from build123d import *

# Parameters (mm, degrees)
ESQUISSE1_W              = 200
ESQUISSE1_H              = 85
BOSS_EXTRU_1_DEPTH       = 30
ENL_V_MAT_EXTRU_3_DEPTH  = 28
ESQUISSE3_W              = 35
ESQUISSE3_H              = 85
ENL_V_MAT_EXTRU_4_DEPTH  = 18
ESQUISSE4_W              = 29.5
ESQUISSE4_H              = 80.5
ENL_V_MAT_EXTRU_5_DEPTH  = 10
CHANFREIN1_SIZE2         = 40
CHANFREIN1_SIZE          = 18
ENL_V_MAT_EXTRU_18_DEPTH = 220.374109685
ENL_V_MAT_EXTRU_19_DEPTH = 220.374109685
CHANFREIN5_SIZE2         = 30
CHANFREIN5_SIZE          = 40
CHANFREIN6_SIZE2         = 25
CHANFREIN6_SIZE          = 40
ESQUISSE10_W             = 40
ESQUISSE10_H             = 2
ENL_V_MAT_EXTRU_20_DEPTH = 2
ENL_V_MAT_EXTRU_21_DEPTH = 4
CONG_6_R                 = 6
CONG_7_R                 = 6
CHANFREIN7_SIZE2         = 119
CHANFREIN7_SIZE          = 2
CHANFREIN8_SIZE          = 0.47
CHANFREIN8_SIZE_2        = 28


# Some blends are built 0.0001 mm under size
with BuildPart() as part:
    # Esquisse1 → Boss.-Extru.1 (new body)
    with BuildSketch(Plane.XY):
        with Locations((100, 42.5)):
            Rectangle(ESQUISSE1_W, ESQUISSE1_H)
    extrude(amount=BOSS_EXTRU_1_DEPTH)

    # Esquisse2 → Enlèv. mat.-Extru.3 (cut)
    with BuildSketch(Plane.XY.offset(30)):
        Polygon((119.192122608, 49.886058148), (121.796845273, 35.113941852), (4.604722665, 14.44980871), (2, 29.221925005), align=None)
    extrude(amount=-ENL_V_MAT_EXTRU_3_DEPTH, mode=Mode.SUBTRACT)

    # Esquisse3 → Enlèv. mat.-Extru.4 (cut)
    with BuildSketch(Plane.XY.offset(30)):
        with Locations((182.5, 42.5)):
            Rectangle(ESQUISSE3_W, ESQUISSE3_H)
    extrude(amount=-ENL_V_MAT_EXTRU_4_DEPTH, mode=Mode.SUBTRACT)

    # Esquisse4 → Enlèv. mat.-Extru.5 (cut)
    with BuildSketch(Plane.XY.offset(12)):
        with Locations((183.25, 42)):
            Rectangle(ESQUISSE4_W, ESQUISSE4_H)
    extrude(amount=-ENL_V_MAT_EXTRU_5_DEPTH, mode=Mode.SUBTRACT)

    # Chanfrein1
    chanfrein1_edges = [part.edges().sort_by_distance(p)[0] for p in [
        (165, 42.5, 30),
    ]]
    chanfrein1_side = [part.faces().sort_by_distance(p)[0] for p in [
        (165, 42.5, 29.64),
    ]]
    chamfer(chanfrein1_edges, length=CHANFREIN1_SIZE - 0.0001, length2=CHANFREIN1_SIZE2 - 0.0001, reference=chanfrein1_side[0])  # a hair under: the kernel refuses the full size

    # Esquisse7 → Enlèv. mat.-Extru.18 (cut, through all)
    with BuildSketch(Plane.XY.offset(30)):
        Polygon((0, 37.959127411), (125, 60), (125, 85), (0, 85), align=None)
    extrude(amount=-ENL_V_MAT_EXTRU_18_DEPTH, mode=Mode.SUBTRACT)

    # Esquisse9 → Enlèv. mat.-Extru.19 (cut, through all)
    with BuildSketch(Plane.XY.offset(30)):
        Polygon((125, 30.113941852), (0, 8.073069264), (0, 0), (125, 0), align=None)
    extrude(amount=-ENL_V_MAT_EXTRU_19_DEPTH, mode=Mode.SUBTRACT)

    # Chanfrein5
    chanfrein5_edges = [part.edges().sort_by_distance(p)[0] for p in [
        (125, 0, 15),
    ]]
    chanfrein5_side = [part.faces().sort_by_distance(p)[0] for p in [
        (125.6, 0, 15),
    ]]
    chamfer(chanfrein5_edges, length=CHANFREIN5_SIZE - 0.0001, length2=CHANFREIN5_SIZE2 - 0.0001, reference=chanfrein5_side[0])  # a hair under: the kernel refuses the full size

    # Chanfrein6
    chanfrein6_edges = [part.edges().sort_by_distance(p)[0] for p in [
        (125, 85, 15),
    ]]
    chanfrein6_side = [part.faces().sort_by_distance(p)[0] for p in [
        (125.5, 85, 15),
    ]]
    chamfer(chanfrein6_edges, length=CHANFREIN6_SIZE - 0.0001, length2=CHANFREIN6_SIZE2 - 0.0001, reference=chanfrein6_side[0])  # a hair under: the kernel refuses the full size

    # Esquisse10 → Enlèv. mat.-Extru.20 (cut)
    with BuildSketch(Plane(origin=(-1.380576153, 7.829636439, 0), x_dir=(0.9848077530122079, 0.17364817766693122, 0), z_dir=(0.17364817766693122, -0.9848077530122079, 0))):
        with Locations((26.401873766, 3)):
            Rectangle(ESQUISSE10_W, ESQUISSE10_H)
    extrude(amount=-ENL_V_MAT_EXTRU_20_DEPTH, mode=Mode.SUBTRACT)

    # Esquisse11 → Enlèv. mat.-Extru.21 (cut)
    with BuildSketch(Plane(origin=(0, 0, 0), x_dir=(-1, 0, 0), z_dir=(0, 0, -1))):
        Polygon((-5, 10.985557391), (-44.39231012, 17.931484498), (-44.045013765, 19.901100004), (-4.652703645, 12.955172897), align=None)
    extrude(amount=-ENL_V_MAT_EXTRU_21_DEPTH, mode=Mode.SUBTRACT)

    # Congé6
    cong_6_edges = [part.edges().sort_by_distance(p)[0] for p in [
        (198, 82.25, 7),
        (198, 1.75, 7),
        (168.5, 1.75, 7),
        (168.5, 82.25, 7),
    ]]
    fillet(cong_6_edges, radius=CONG_6_R)

    # Congé7
    cong_7_edges = [part.edges().sort_by_distance(p)[0] for p in [
        (200, 85, 6),
        (200, 0, 6),
    ]]
    fillet(cong_7_edges, radius=CONG_7_R)

    # Chanfrein7
    chanfrein7_edges = [part.edges().sort_by_distance(p)[0] for p in [
        (120.494483941, 42.5, 2),
    ]]
    chanfrein7_side = [part.faces().sort_by_distance(p)[0] for p in [
        (120.494483941, 42.5, 2.04),
    ]]
    chamfer(chanfrein7_edges, length=CHANFREIN7_SIZE - 0.0001, length2=CHANFREIN7_SIZE2 - 0.0001, reference=chanfrein7_side[0])  # a hair under: the kernel refuses the full size

    # Chanfrein8
    # the kernel refuses this chamfer: 28, 0.47 mm, written as the material it adds along each edge
    with BuildSketch(Plane(origin=(17.246244149, -57.243822257, 2), x_dir=(0.3939624540892155, 0.06946621004204875, -0.9164976979951431), z_dir=(-0.1736481776669307, 0.984807753012208, 0))) as chanfrein8_piece_1_section:
        Polygon((CHANFREIN8_SIZE * 0.400039959966, -CHANFREIN8_SIZE * 0.916497697995), (-CHANFREIN8_SIZE_2 * 0.916497697995, -CHANFREIN8_SIZE_2 * 0.400039959966), (0, 0), align=None)
    chanfrein8_piece_1 = extrude(amount=160.599241573, mode=Mode.PRIVATE)
    chanfrein8_piece_1 = split(chanfrein8_piece_1, bisect_by=Plane(origin=(0.668634618, 38.077025735, 2.989674186), z_dir=(0.17364817766693805, -0.9848077530122068, 0)), keep=Keep.TOP, mode=Mode.PRIVATE)
    chanfrein8_piece_1 = split(chanfrein8_piece_1, bisect_by=Plane(origin=(5.084858853, 13.03137352, 2.989674186), z_dir=(-0.17364817766693125, 0.9848077530122079, 0)), keep=Keep.TOP, mode=Mode.PRIVATE)
    add(chanfrein8_piece_1)


solid = part.part
Read the model definition and answer for the solid it produces. Units are mm, in the model's axes. A direction names the side the tool comes from. Coordinates: 2 decimals unless noted, no trailing zeros. Write each loop counter-clockwise with the first axis right and the second up, starting at its lowest first coordinate (ties: lowest second). Pieces come first, ordered by that corner, then holes. Notation, with made-up numbers: (35, 43.25) - (54, 43.25) arc R14 ccw to (54, 70.25) - close; hole circle Ø3 at (67.5, 17). An arc over 180 degrees is marked (long way). One line per question, with ' | ' between items.
Q1. Find section B-B, the plane z = 10. State how many separate pieces and enclosed holes the cut face has, plus the area to 3 significant figures.
Result set:
separate pieces: 1 | enclosed holes: 2 | area: 4,870 mm^2
Q2. For faces 4 (the flat face through (24.625, 16.477, 1.972)), 5 (the flat face through (183, 43, 2)), 6 (the flat face through (63.375, 19.248, 15.21)), 7 (the flat face through (179, 85, 6)), determine the directions among +Z, -Z, +X, -X, +Y, -Y from which every point of the face is accessible in a straight line to the end or side of a thin tool.
Result set:
face 4: -Z | face 5: +Z | face 6: +Z, -Z, -Y | face 7: +Z, -Z, +X, -X, +Y
Q3. Find section A-A, the plane x = 18. Write down the section's boundary in (y, z).
Result set:
outline: (11.25, 0) - (13.28, 0) - (13.28, 2) - (11.25, 2) - close; (11.25, 4) - (15.31, 4) - (15.31, 0) - (41.13, 0) - (41.13, 30) - (32.04, 30) - (32.04, 2.27) - (16.81, 2.23) - (16.81, 30) - (11.25, 30) - close
Q4. Each of these flat-tipped pins is pushed along its axis until it touches: P1, Ø10.5, axis at x = 174.5, y = 51, coming from the +Z side; P2, Ø1, axis at x = 161.5, y = 43, coming from the -Z side; P3, Ø1, axis at y = 65.5, z = 17.5, coming from the +X side. Where does it stop, or does it pass through?
Result set:
P1: z = 2 | P2: z = 0 | P3: x = 153.89
Q5. Determine the mould class of faces 1 (the flat face through (121, 43, 0)), 2 (the flat face through (140.28, 69.55, 11.88)), 3 (the flat face through (24, 13, 2)) for opening direction X: +X half, -X half, draft (parallel to the pull), parting line (faces both ways), or undercut.
Result set:
face 1: draft | face 2: -X half | face 3: undercut
Q6. Consider L1, parallel to Z at x = 177, y = 71; L2, parallel to Y at x = 55, z = 8.5; L3, parallel to Y at x = 35, z = 19. Determine where each line is inside the solid, lowest interval first. Write a range as [from, to].
Result set:
L1: [0, 2] | L2: [17.77, 23.34], [38.57, 47.66] | L3: [14.24, 19.81], [35.04, 44.13]
